CAD build for the part. Positions are in the model's coordinates, mm. Give positions to 0.01 mm unless a question says otherwise; leave off trailing zeros. Order: outer loops, then holes, each group sorted by start corner. A loop starts at its lowest first (then second) coordinate and runs counter-clockwise, first axis right, second up.
Item 1: Band-saw the part on A-A on y = -5. Give the cut face in (x, z).
Item 2: Wall check: L1, parallel to Y at x = 5, z = 2.6; L2, parallel to X at y = 0.25, z = 2.05; L3, parallel to Y at x = 0.75, z = 1.7. Give the ranges that are in metal, low to high.
Item 3: Band-saw the part on B-B on x = -3.75. Give the cut face in (y, z), plus the area to 3 significant figures.
Item 4: Flat gauge pin, fed straight in: P1, Ø1, axis at x = 1.5, z = 2.5, coming from the +Y side. Where does the tip first touch, or does it go through?
```python
from build123d import *

# Parameters (mm, degrees)
F0_W     = 12.7
F0_H     = 12.7
F1_DEPTH = 3.18
F3_DEPTH = 12.701
F5_DEPTH = 6.5
F6_R     = 0.8
F7_ANGLE = 45


with BuildPart() as f1:
    # F0 (on Top) → F1 (new body)
    with BuildSketch(Plane.XY):
        Rectangle(F0_W, F0_H)
    extrude(amount=F1_DEPTH)

    # F2 (on face) → F3 (cut, through all)
    with BuildSketch(Plane.XZ.offset(6.35)):
        Polygon((6.35, 0), (6.35, 3.18), (5.7318706169, 0), align=None)
        Polygon((-5.7318706169, 0), (-6.35, 3.18), (-6.35, 0), align=None)
    extrude(amount=-F3_DEPTH, mode=Mode.SUBTRACT)

    # F4 (on Right) → F5 (cut, symmetric)
    with BuildSketch(Plane.YZ):
        Polygon((6.35, 0), (6.35, 3.18), (5.7318706169, 0), align=None)
        Polygon((-5.7318706169, 0), (-6.35, 3.18), (-6.35, 0), align=None)
    extrude(amount=F5_DEPTH, both=True, mode=Mode.SUBTRACT)

    # F6
    f6_edges = [f1.edges().sort_by_distance(p)[0] for p in [
        (6.040935, -6.040935, 1.59),
        (-6.040935, -6.040935, 1.59),
        (6.040935, 6.040935, 1.59),
        (-6.040935, 6.040935, 1.59),
    ]]
    fillet(f6_edges, radius=F6_R)


with BuildPart() as f1_1:
    # F7: moved
    add(f1.part.rotate(Axis((0, 0, 0.6975659635), (0, 0, 1)), F7_ANGLE))


solid = f1_1.part
```
The answers:
1. outline: (-3.98, 3.18) - (-3.11, 0) - (3.11, 0) - (3.98, 3.18) - close
2. L1: y = -3.82 to 3.82
2. L2: x = -8.31 to 8.31
2. L3: y = -7.82 to 7.82
3. outline: (-5.23, 3.18) - (-4.36, 0) - (4.36, 0) - (5.23, 3.18) - close
3. area: 30.5 mm2
4. P1: stops at y = 7.81
